Can you work these out from the drawing? Everything is in mm from the part's minimum corner. A direction names the side the tool comes from. Round coordinates to 2 decimals unless told otherwise and drop trailing zeros. Write each loop counter-clockwise with the first axis right and the second up, starting at its lowest first coordinate (ties: lowest second). Pieces come first, ordered by that corner, then holes. Notation, with made-up numbers: (68.25, 69) - (72.25, 69) arc R7 ccw to (72.25, 74) - close; hole circle Ø9 at (-14.5, -16.5). An arc over 180 degrees is marked (long way). One line per item, written item: value. Start each with the question number.
Item 1: Imagine slicing it at A-A, the plane x = 2.25. Please give me the cut outline in (y, z), then the cut area to 3 significant figures.
Item 2: If I drill on line 1 (Y direction, x = 16.5, z = 0.2); line 2 (Y direction, x = 2.25, z = 0.8); line 3 (Y direction, x = 19, z = 0.55), over which ranges is the centre line in solid material (lowest first)?
Item 3: Imagine slicing it at C-C, the plane y = 13.5. Please give me the cut outline in (x, z).
Item 4: Imagine slicing it at B-B, the plane z = 0.65. Count the separate pieces of the cut face and the enclosed holes in it, then the cut area to 3 significant figures.
Item 5: For P1, Ø1.1, axis at y = 12.5, z = 2, coming from the -X side; P2, Ø1.2, axis at x = 15, z = 2.5, coming from the +Y side; P3, Ø1.3, axis at x = 10, y = 2.5, coming from the +Z side; P4, Ø0.5, axis at y = 12.5, z = 2.5, coming from the +X side, each with a flat end and sliding along its axis, tell me the tip position at first contact or that it passes through.
Item 6: Thinking about a two-plate mould opening in Y: for the marked faces 3, 4 and 5, which applies, released by +Y, released by -Y, zero draft, split by the parting line, or undercut?
Item 7: For the marked faces 1 and 2, which set-ups out of +Z, -Z, +X, -X, +Y, -Y let a thin tool reach every point of the face, with its end or its side?
Item 8: Imagine slicing it at D-D, the plane z = 2.5. Please give me the cut outline in (x, y).
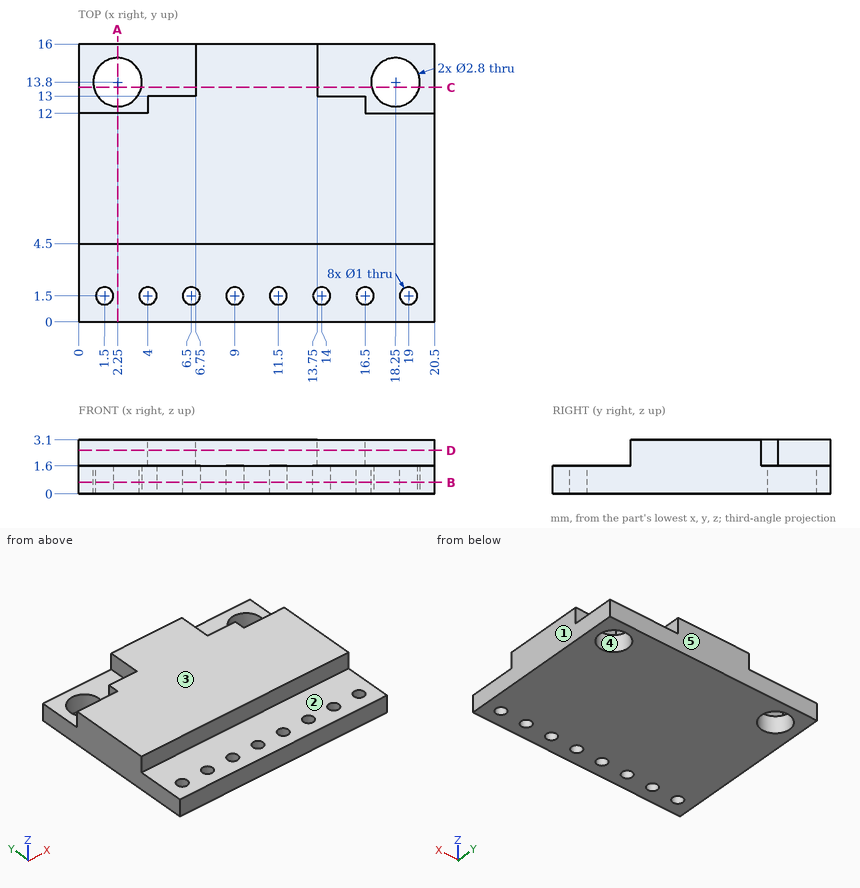
Values follow:
1. outline: (0, 0) - (12.4, 0) - (12.4, 1.6) - (12, 1.6) - (12, 3.1) - (4.5, 3.1) - (4.5, 1.6) - (0, 1.6) - close; (15.2, 0) - (16, 0) - (16, 1.6) - (15.2, 1.6) - close
1. area: 32.4 mm^2
2. line 1: y = 0 to 1, 2 to 16
2. line 2: y = 0 to 12.4, 15.2 to 16
2. line 3: y = 0 to 1, 2 to 12.62, 14.98 to 16
3. outline: (0, 0) - (0.88, 0) - (0.88, 1.6) - (0, 1.6) - close; (3.62, 0) - (16.88, 0) - (16.88, 1.6) - (13.75, 1.6) - (13.75, 3.1) - (6.75, 3.1) - (6.75, 1.6) - (3.62, 1.6) - close; (19.62, 0) - (20.5, 0) - (20.5, 1.6) - (19.62, 1.6) - close
4. separate pieces: 1
4. enclosed holes: 10
4. area: 309 mm^2
5. P1: stops at x = 0
5. P2: stops at y = 13
5. P3: stops at z = 1.6
5. P4: stops at x = 16.5
6. face 3: zero draft
6. face 4: undercut
6. face 5: released by +Y
7. face 1: +Z, -Z, +X, +Y, -Y
7. face 2: +Z, +X, -X, -Y
8. outline: (0, 4.5) - (20.5, 4.5) - (20.5, 12) - (16.5, 12) - (16.5, 13) - (13.75, 13) - (13.75, 16) - (6.75, 16) - (6.75, 13) - (4, 13) - (4, 12) - (0, 12) - close
